Could you check a few things on this model? Use its own coordinates, in mm. Face numbers are marked on the shaded views. A direction names the side the tool comes from. Coordinates: 2 decimals unless noted, no trailing zeros. Loops run counter-clockwise (first coordinate to the right, second up) from the corner with the lowest first, then second, coordinate; pieces in that order, holes last. Notation, with made-up numbers: M 56,69.5 L 84,69.5 A37 cw 84,105.5 Z; hole C -36.5,22.5 d8. An arc over 180 degrees is marked long. Write each question's results on one line, items separated by ' | '.
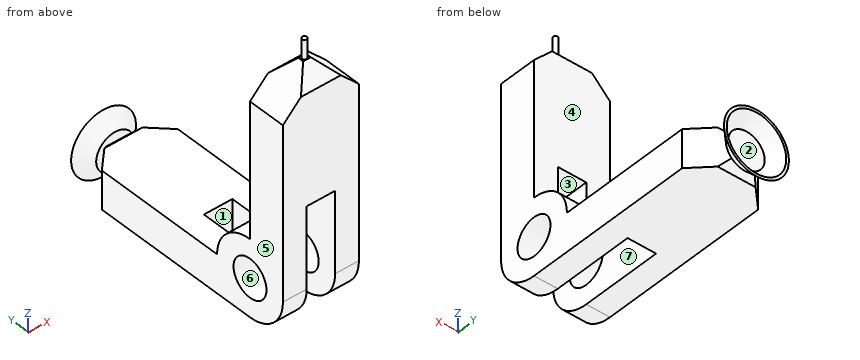
```python
from build123d import *

# Parameters (mm, degrees)
SKETCH1_TOOL_TIP_R  = 10
BOSS_EXTRUDE1_DEPTH = 20
CHAMFER1_SIZE       = 18
CUT_EXTRUDE1_DEPTH  = 7.5
SKETCH3_TOOL_TIP_R  = 1.25
BOSS_EXTRUDE2_DEPTH = 10
CHAMFER2_SIZE       = 15


with BuildPart() as part:
    # sketch1_tool_tip → Boss-Extrude1 (new body, symmetric)
    with BuildSketch(Plane(origin=(0, 0, 0), x_dir=(0, 0, -1), z_dir=(1, 0, 0))):
        with BuildLine():
            Line((-100, 0), (-108.5, -8.5))
            Line((-108.5, -8.5), (-108.5, -11.5))
            Line((-108.5, -11.5), (-100, -20))
            Line((-100, -20), (0, -20))
            ThreePointArc((0, -20), (14.142135624, -14.142135624), (20, 0))
            Line((20, 0), (20, 100))
            Line((20, 100), (15, 105))
            Line((15, 105), (5, 105))
            Line((5, 105), (0, 100))
            Line((0, 100), (0, 20))
            ThreePointArc((0, 20), (-14.142135624, 14.142135624), (-20, 0))
            Line((-20, 0), (-100, 0))
        make_face()
        Circle(SKETCH1_TOOL_TIP_R, mode=Mode.SUBTRACT)
    extrude(amount=BOSS_EXTRUDE1_DEPTH, both=True)

    # Chamfer1
    chamfer1_edges = [part.edges().sort_by_distance(p)[0] for p in [
        (-20, -10, 108.5),
        (20, -10, 108.5),
    ]]
    chamfer(chamfer1_edges, length=CHAMFER1_SIZE)

    # sketch2_tool_tip → Cut-Extrude1 (cut, symmetric)
    with BuildSketch(Plane(origin=(0, 0, 0), x_dir=(0, 0, -1), z_dir=(1, 0, 0))):
        with BuildLine():
            Line((-42.42, -20), (0, -20))
            ThreePointArc((0, -20), (14.142135624, -14.142135624), (20, 0))
            Line((20, 0), (20, 42.42))
            Line((20, 42.42), (0, 42.42))
            Line((0, 42.42), (0, 20))
            ThreePointArc((0, 20), (-14.142135624, 14.142135624), (-20, 0))
            Line((-20, 0), (-42.42, 0))
            Line((-42.42, 0), (-42.42, -20))
        make_face()
    extrude(amount=CUT_EXTRUDE1_DEPTH, both=True, mode=Mode.SUBTRACT)

    # sketch3_tool_tip → Boss-Extrude2 (add)
    with BuildSketch(Plane.XY.offset(108.5)):
        with Locations((0, -10)):
            Circle(SKETCH3_TOOL_TIP_R)
    extrude(amount=BOSS_EXTRUDE2_DEPTH)

    # Chamfer2
    chamfer2_edges = [part.edges().sort_by_distance(p)[0] for p in [
        (-20, 105, -10),
        (20, 105, -10),
    ]]
    chamfer(chamfer2_edges, length=CHAMFER2_SIZE)

    # sketch4_tool_tip → Revolve1 (revolve)
    with BuildSketch(Plane(origin=(0, 0, -10), x_dir=(-1, 0, 0), z_dir=(0, 0, -1))):
        Polygon((0, 105), (10, 105), (17.071067812, 112.071067812), (15.656854249, 112.071067812), (9.585786438, 106), (0, 106), align=None)
    revolve(axis=Axis((0, 105, -10), (0, -1, 0)))


solid = part.part
```
(1) Imagine slicing it at A-A, the plane z = 24.5. List the corners of the cut face in (x, y) for me.
Reported:
outline: M -20,-20 L -7.5,-20 L -7.5,0 L -20,0 Z; M 7.5,-20 L 20,-20 L 20,0 L 7.5,0 Z
(2) If we mould it in two halves opening along X, with no side actions, what happens to the marked faces 5, 6 and 7? For each: released by +X, released by -X, zero draft, split by the parting line, or undercut.
Reported:
face 5: released by -X | face 6: zero draft | face 7: undercut
(3) Which directions (+Z, -Z, +X, -X, +Y, -Y) give clear straight access to the entire face, cutting with the end or side of a thin tool? Please do the marked faces 1, 2, 3 and 4.
Reported:
face 1: +Z, -Z, -Y | face 2: +Y | face 3: -Z, +Y, -Y | face 4: +Z, +X, -X, +Y
(4) Imagine slicing it at C-C, the plane z = 45. List the corners of the cut face in (x, y) for me, and give its area (3 significant figures).
Reported:
outline: M -20,-20 L 20,-20 L 20,0 L -20,0 Z | area: 800 mm2
(5) Will these pins go through, and if not, where does the flat tip stop? P1, Ø1.5, axis at x = 10.5, z = 44.5, coming from the +Y side; P2, Ø7.5, axis at x = 1, y = -12, coming from the -Z side; P3, Ø5, axis at x = -11.5, y = 69.5, coming from the +Z side.
Reported:
P1: stops at y = 0 | P2: stops at z = 42.42 | P3: stops at z = 0
(6) Please list where these lines run through material, in increasing order: probe 1 along X at (y, z) = (13.5, 0.5); probe 2 along Z at (x, y) = (-16, 91). Write a range as from..to.
Reported:
probe 1: x = -20..-7.5, 7.5..20 | probe 2: z = -20..0
(7) Imagine slicing it at B-B, the plane y = 16.5. List the corners of the cut face in (x, z) for me, and give its area (3 significant figures).
Reported:
outline: M -20,-20 L -7.5,-20 L -7.5,11.3 L -20,11.3 Z; M 7.5,-20 L 20,-20 L 20,11.3 L 7.5,11.3 Z | area: 783 mm2
